Source: three-view drawing plus pictorial views. Frame: mm from the lowest corner of the part. A direction names the side the tool comes from. Round coordinates to 2 decimals unless told otherwise and drop trailing zeros. Loops run counter-clockwise (first coordinate to the right, second up) from the corner with the lowest first, then second, coordinate; pieces in that order, holes last. Notation, with made-up numbers: (-35.5, -33.75) -> (-24.5, -33.75) arc R13 ccw to (-24.5, -21.75) -> close; hole circle Ø6 at (38.5, -28). An arc over 180 degrees is marked (long way). Answer in a Markdown table with one row per item. Add a question column.
Q1. Section A-A, the plane y = 13.5. Output: boundary loops of the cut face in (x, z), and give its area (3 significant figures).
Q2. Reachability of the marked faces 1 and 2 from +Z, -Z, +X, -X, +Y, -Y: full face, straight path, thin tool, end or side. Return the list, or none.
Q3. Section B-B, the plane y = 8.75. Output: boundary loops of the cut face in (x, z), and give its area (3 significant figures).
Q4. Pin query (flat end, axial travel): pin 1 (1 mm diameter, centred on x = 1, z = 1.5, fed in from +Y); pin 2 (1.5 mm diameter, centred on y = 14, z = 5, fed in from +X); pin 3 (1.5 mm diameter, centred on x = 5, y = 3.5, fed in from +Z). Return the tip coordinate at first contact, or that it passes through.
Q5. Ray query, L1, parallel to Y at x = 4, z = 4.2; L2, parallel to Y at x = 4.75, z = 4.6; L3, parallel to X at y = 6.25, z = 1.7. Return the intervals inside material, ascending. Write a range as from..to.
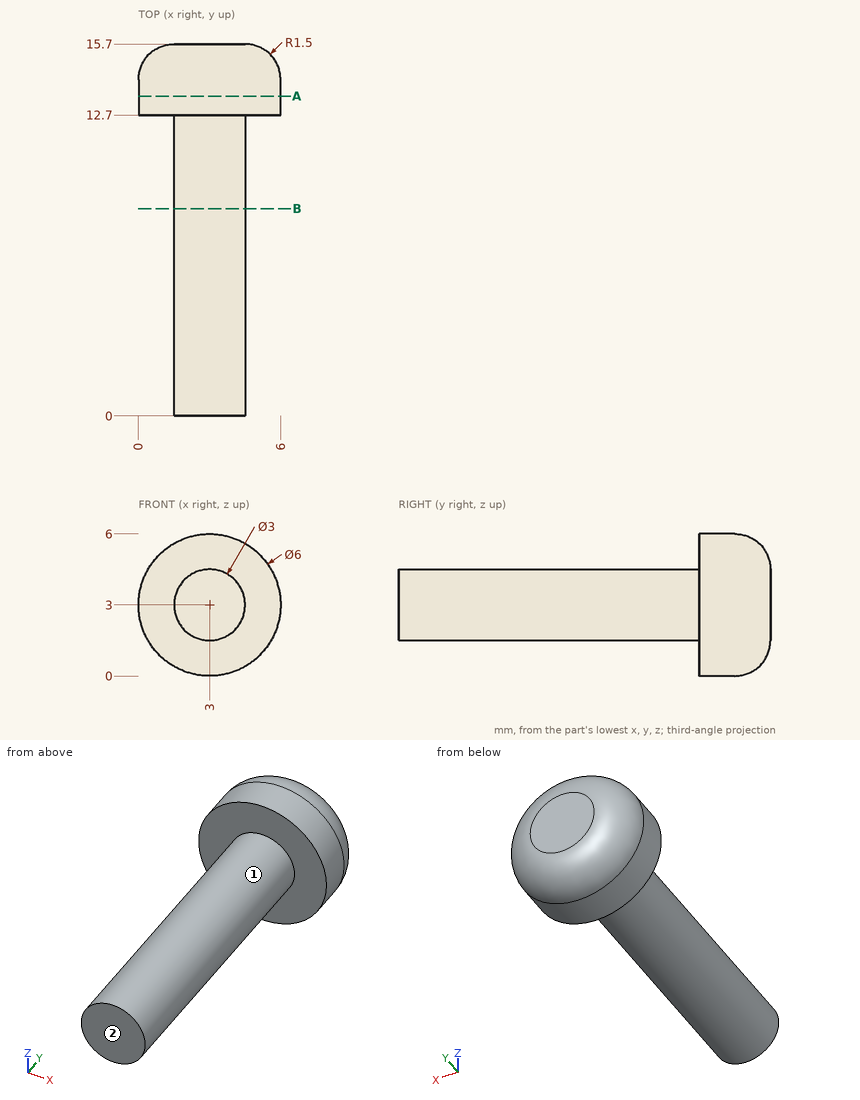
Answer block:
| question | item | result |
|---|---|---|
| 1 | outline | circle Ø6 at (3, 3) |
| 1 | area | 28.3 mm^2 |
| 2 | face 1 | -Y |
| 2 | face 2 | +Z, -Z, +X, -X, -Y |
| 3 | outline | circle Ø3 at (3, 3) |
| 3 | area | 7.07 mm^2 |
| 4 | pin 1 | y = 15.61 |
| 4 | pin 2 | x = 5.73 |
| 4 | pin 3 | z = 3.83 |
| 5 | L1 | 12.7..15.7 |
| 5 | L2 | 12.7..15.42 |
| 5 | L3 | 2.25..3.75 |
